Could you check a few things on this model? Use its own coordinates, in mm. Face numbers are marked on the shaded views. A direction names the side the tool comes from. Coordinates: 2 decimals unless noted, no trailing zeros. Loops run counter-clockwise (first coordinate to the right, second up) from the corner with the lowest first, then second, coordinate; pieces in that order, holes last. Notation, with made-up numbers: M -23,-16.75 L 3,-16.75 A23 ccw 3,1.25 Z; hole C 20.5,27 d11. An arc over 180 degrees is marked long. Write each question's results on one line, items separated by ' | '.
```python
from build123d import *

# Parameters (mm, degrees)
SKETCH1_R           = 17.5
BOSS_EXTRUDE1_DEPTH = 63
SKETCH2_R           = 12.5
BOSS_EXTRUDE2_DEPTH = 6
FILLET1_R           = 1


with BuildPart() as part:
    # Sketch1 → Boss-Extrude1 (new body)
    with BuildSketch(Plane.XY):
        Circle(SKETCH1_R)
    extrude(amount=BOSS_EXTRUDE1_DEPTH)

    # Sketch2 → Boss-Extrude2 (add)
    with BuildSketch(Plane(origin=(0, 0, 0), x_dir=(-1, 0, 0), z_dir=(0, 0, -1))):
        with Locations(Location((0, 0, 0), (0, 0, 180))):
            Circle(SKETCH2_R)
    extrude(amount=BOSS_EXTRUDE2_DEPTH)

    # Fillet1
    fillet1_edges = [part.edges().sort_by_distance(p)[0] for p in [
        (-17.5, 0, 0),
        (-17.5, 0, 63),
    ]]
    fillet(fillet1_edges, radius=FILLET1_R)


solid = part.part
```
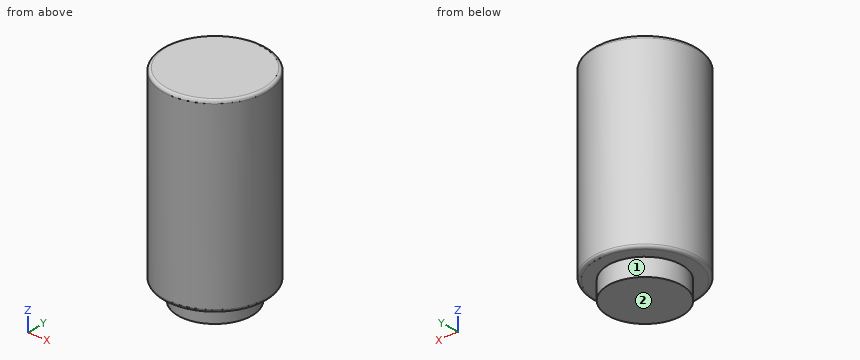
(1) Imagine slicing it at A-A, the plane y = 0. List the corners of the cut face in (x, z) for me, and give its area (3 significant figures).
Reported:
outline: M -17.5,1 A1 ccw -16.5,0 L -12.5,0 L -12.5,-6 L 12.5,-6 L 12.5,0 L 16.5,0 A1 ccw 17.5,1 L 17.5,62 A1 ccw 16.5,63 L -16.5,63 A1 ccw -17.5,62 Z | area: 2,350 mm2
(2) Imagine slicing it at C-C, the plane z = 53.5. List the corners of the cut face in (x, y) for me, and give its area (3 significant figures).
Reported:
outline: C 0,0 d35 | area: 962 mm2
(3) Imagine slicing it at D-D, the plane z = -1. List the corners of the cut face in (x, y) for me.
Reported:
outline: C 0,0 d25
(4) Will these pins go through, and if not, where does the flat tip stop? P1, Ø12, axis at y = -10.5, z = 50.5, coming from the +X side; P2, Ø8, axis at y = -3, z = 13, coming from the -X side; P3, Ø6, axis at y = -7, z = 30.5, coming from the +X side; P4, Ø4, axis at y = -10.5, z = 49, coming from the -X side.
Reported:
P1: stops at x = 16.91 | P2: stops at x = -17.5 | P3: stops at x = 17.04 | P4: stops at x = -15.3
(5) Please list where these lines run through material, in increasing order: probe 1 along Z at (x, y) = (-14, 6.5); probe 2 along X at (y, z) = (0.5, 51); probe 3 along X at (y, z) = (8, 12.5). Write a range as from..to.
Reported:
probe 1: z = 0..63 | probe 2: x = -17.49..17.49 | probe 3: x = -15.56..15.56
(6) Which directions (+Z, -Z, +X, -X, +Y, -Y) give clear straight access to the entire face, cutting with the end or side of a thin tool? Please do the marked faces 1 and 2.
Reported:
face 1: -Z | face 2: -Z, +X, -X, +Y, -Y
